Read the model definition and answer for the solid it produces. Units are mm, in the model's axes. A direction names the side the tool comes from. Coordinates: 2 decimals unless noted, no trailing zeros. Loops run counter-clockwise (first coordinate to the right, second up) from the corner with the lowest first, then second, coordinate; pieces in that order, holes last. Notation, with made-up numbers: (51, 23) -> (85, 23) arc R25 cw to (85, 52) -> close; hole circle Ø10 at (36, 67). An arc over 180 degrees is marked (long way). Answer in a Markdown table with one row per item.
```python
from build123d import *

# Parameters (mm, degrees)
SKETCH_1_W              = 36
SKETCH_1_H              = 36
EXTRUDE_1_DEPTH         = 11
SKETCH_2_W              = 24.5
SKETCH_2_H              = 24.5
EXTRUDE_2_DEPTH         = 2.5
SKETCH_3_R              = 7
EXTRUDE_3_DEPTH         = 15
HOLE_WIZARD_2_5_2_5_1_D = 2.5


with BuildPart() as part:
    # 草图1 → 凸台-拉伸1 (new body)
    with BuildSketch(Plane.XY):
        Rectangle(SKETCH_1_W, SKETCH_1_H)
    extrude(amount=EXTRUDE_1_DEPTH)

    # 草图2 → 凸台-拉伸2 (add)
    with BuildSketch(Plane.XY.offset(11)):
        Rectangle(SKETCH_2_W, SKETCH_2_H)
    extrude(amount=EXTRUDE_2_DEPTH)

    # 草图3 → 凸台-拉伸3 (add)
    with BuildSketch(Plane.XY.offset(13.5)):
        Circle(SKETCH_3_R)
    extrude(amount=EXTRUDE_3_DEPTH)

    # Ø2.5 (2.5) 直径孔1 (through all)
    with Locations(Plane(origin=(18, 0, 0), x_dir=(0, 0, -1), z_dir=(1, 0, 0))):
        with Locations((-5.5, 0)):
            Hole(HOLE_WIZARD_2_5_2_5_1_D / 2)


solid = part.part
```
1. A cutting plane is placed at C-C on x = 0. Give the vertices of the cut face in (y, z).
A:
| item | result |
|---|---|
| outline | (-18, 0) -> (18, 0) -> (18, 11) -> (12.25, 11) -> (12.25, 13.5) -> (7, 13.5) -> (7, 28.5) -> (-7, 28.5) -> (-7, 13.5) -> (-12.25, 13.5) -> (-12.25, 11) -> (-18, 11) -> close; hole circle Ø2.5 at (0, 5.5) |
2. The mould has two halves that part along Y. Classify faces 4 (the cylindrical face through (-0.25, 0.05, 4.25)), 5 (the flat face through (0, 18, 5)), 6 (the flat face through (-18, 0, 4)): pulls with the +Y half, pulls with the -Y half, needs draft (parallel to the pull), parting line crosses it, or undercut.
A:
| item | result |
|---|---|
| face 4 | undercut |
| face 5 | pulls with the +Y half |
| face 6 | needs draft |
3. A cutting plane is placed at B-B on y = 0. Give the vertices of the cut face in (x, z).
A:
| item | result |
|---|---|
| outline | (-18, 0) -> (18, 0) -> (18, 4.25) -> (-18, 4.25) -> close; (-18, 6.75) -> (18, 6.75) -> (18, 11) -> (12.25, 11) -> (12.25, 13.5) -> (7, 13.5) -> (7, 28.5) -> (-7, 28.5) -> (-7, 13.5) -> (-12.25, 13.5) -> (-12.25, 11) -> (-18, 11) -> close |
4. A cutting plane is placed at D-D on y = -13. Give the vertices of the cut face in (x, z), and give its area (3 significant figures).
A:
| item | result |
|---|---|
| outline | (-18, 0) -> (18, 0) -> (18, 11) -> (-18, 11) -> close |
| area | 396 mm2 |
5. Given pin 1 Ø2 at (x, y) = (2, -11.5) entering from +Z; pin 2 Ø0.8 at (x, z) = (4, 12.5) entering from +Y; pin 3 Ø12 at (x, z) = (10, 24) entering from -Y, each flat-ended and moving along its own axis, determine where each tip first touches the part or whether it passes through.
A:
| item | result |
|---|---|
| pin 1 | stops at z = 13.5 |
| pin 2 | stops at y = 12.25 |
| pin 3 | stops at y = -5.74 |
6. A tool of negligible diameter and unlimited length cuts with its end or side. For faces 1 (the flat face through (12.25, 0, 12)), 2 (the cylindrical face through (6.466, -2.681, 20.895)), 3 (the flat face through (-12.25, 0, 12)), from which of +Z, -Z, +X, -X, +Y, -Y can it reach the whole face along a straight path? Write none if from no direction.
A:
| item | result |
|---|---|
| face 1 | +Z, +X, +Y, -Y |
| face 2 | +Z |
| face 3 | +Z, -X, +Y, -Y |
7. Find the intervals of material crossed by probe 1 along Y at (x, z) = (-5, 5.5); probe 2 along X at (y, z) = (10.5, 12.5); probe 3 along Z at (x, y) = (5.5, -6), in increasing order.
A:
| item | result |
|---|---|
| probe 1 | y = -18 to -1.25, 1.25 to 18 |
| probe 2 | x = -12.25 to 12.25 |
| probe 3 | z = 0 to 13.5 |
8. A cutting plane is placed at A-A on z = 5.5. Give the vertices of the cut face in (x, y).
A:
| item | result |
|---|---|
| outline | (-18, -18) -> (18, -18) -> (18, -1.25) -> (-18, -1.25) -> close; (-18, 1.25) -> (18, 1.25) -> (18, 18) -> (-18, 18) -> close |
